Check sheet for the modelled part. Datum: model origin and axes. Units: mm. Give positions to 0.01 mm unless a question says otherwise; leave off trailing zeros. Write each loop counter-clockwise with the first axis right and the second up, starting at its lowest first coordinate (ties: lowest second). Pieces come first, ordered by that corner, then holes. Notation, with made-up numbers: (86, 72) -> (93, 72) arc R14 ccw to (93, 96) -> close; hole circle Ø9 at (31, -1). An arc over 180 degrees is marked (long way). Answer as a JSON object with one key per item and string values.
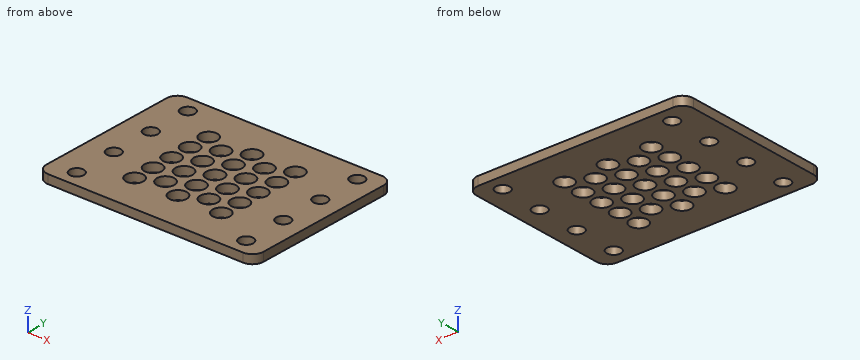
from build123d import *

# Parameters (mm, degrees)
SKETCH_W     = 100
SKETCH_H     = 75
SKETCH_R     = 3.2
PAD_DEPTH    = 4
SKETCH001_R  = 4
POCKET_DEPTH = 5
FILLET_R     = 5


with BuildPart() as part:
    # Sketch → Pad (new body)
    with BuildSketch(Plane.XY):
        with Locations((50, 37.5)):
            Rectangle(SKETCH_W, SKETCH_H)
        with Locations((11.871567, 67.5)):
            Circle(SKETCH_R, mode=Mode.SUBTRACT)
        with Locations((11.871567, 47.5)):
            Circle(SKETCH_R, mode=Mode.SUBTRACT)
        with Locations((11.871567, 27.5)):
            Circle(SKETCH_R, mode=Mode.SUBTRACT)
        with Locations((11.871567, 7.5)):
            Circle(SKETCH_R, mode=Mode.SUBTRACT)
        with Locations((90, 67.5)):
            Circle(SKETCH_R, mode=Mode.SUBTRACT)
        with Locations((90, 47.5)):
            Circle(SKETCH_R, mode=Mode.SUBTRACT)
        with Locations((90, 27.5)):
            Circle(SKETCH_R, mode=Mode.SUBTRACT)
        with Locations((90, 7.5)):
            Circle(SKETCH_R, mode=Mode.SUBTRACT)
    extrude(amount=PAD_DEPTH)

    # Sketch001 (on Face14 of Pad) → Pocket (cut)
    with BuildSketch(Plane.XY.offset(4)):
        with Locations((30, 57.5)):
            Circle(SKETCH001_R)
        with Locations((30, 47.5)):
            Circle(SKETCH001_R)
        with Locations((30, 37.5)):
            Circle(SKETCH001_R)
        with Locations((30, 27.5)):
            Circle(SKETCH001_R)
        with Locations((30, 17.5)):
            Circle(SKETCH001_R)
        with Locations((50, 57.5)):
            Circle(SKETCH001_R)
        with Locations((50, 47.5)):
            Circle(SKETCH001_R)
        with Locations((50, 37.5)):
            Circle(SKETCH001_R)
        with Locations((50, 27.5)):
            Circle(SKETCH001_R)
        with Locations((50, 17.5)):
            Circle(SKETCH001_R)
        with Locations((70, 57.5)):
            Circle(SKETCH001_R)
        with Locations((70, 47.5)):
            Circle(SKETCH001_R)
        with Locations((70, 37.5)):
            Circle(SKETCH001_R)
        with Locations((70, 27.5)):
            Circle(SKETCH001_R)
        with Locations((70, 17.5)):
            Circle(SKETCH001_R)
        with Locations((40, 52.5)):
            Circle(SKETCH001_R)
        with Locations((40, 42.5)):
            Circle(SKETCH001_R)
        with Locations((40, 32.5)):
            Circle(SKETCH001_R)
        with Locations((40, 22.5)):
            Circle(SKETCH001_R)
        with Locations((60, 52.5)):
            Circle(SKETCH001_R)
        with Locations((60, 42.5)):
            Circle(SKETCH001_R)
        with Locations((60, 32.5)):
            Circle(SKETCH001_R)
        with Locations((60, 22.5)):
            Circle(SKETCH001_R)
    extrude(amount=-POCKET_DEPTH, mode=Mode.SUBTRACT)

    # Fillet
    fillet_edges = [part.edges().sort_by_distance(p)[0] for p in [
        (100, 75, 2),
        (100, 0, 2),
        (0, 75, 2),
        (0, 0, 2),
    ]]
    fillet(fillet_edges, radius=FILLET_R)


solid = part.part
1. Sectioned sample at A-A, the plane x = 60. Enter the section's corners in (y, z).
Determined:
{"outline": "(0, 0) -> (18.5, 0) -> (18.5, 4) -> (0, 4) -> close; (26.5, 0) -> (28.5, 0) -> (28.5, 4) -> (26.5, 4) -> close; (36.5, 0) -> (38.5, 0) -> (38.5, 4) -> (36.5, 4) -> close; (46.5, 0) -> (48.5, 0) -> (48.5, 4) -> (46.5, 4) -> close; (56.5, 0) -> (75, 0) -> (75, 4) -> (56.5, 4) -> close"}
2. Go/stop test with a flat-tipped pin: P1, Ø9, axis at x = 60, y = 22.5, coming from the +Z side. Record where the tip stops, or that it passes through.
Determined:
{"P1": "z = 4"}
3. Sectioned sample at B-B, the plane y = 67.5. Enter the section's corners in (x, z).
Determined:
{"outline": "(0, 0) -> (8.67, 0) -> (8.67, 4) -> (0, 4) -> close; (15.07, 0) -> (86.8, 0) -> (86.8, 4) -> (15.07, 4) -> close; (93.2, 0) -> (100, 0) -> (100, 4) -> (93.2, 4) -> close"}
4. Scan lines: L1, parallel to Y at x = 70, z = 2.1; L2, parallel to Y at x = 90, z = 1.6; L3, parallel to Y at x = 60, z = 2.1. Record each from-to range of solid material in increasing order. Write a range as [from, to].
Determined:
{"L1": "[0, 13.5], [21.5, 23.5], [31.5, 33.5], [41.5, 43.5], [51.5, 53.5], [61.5, 75]", "L2": "[0, 4.3], [10.7, 24.3], [30.7, 44.3], [50.7, 64.3], [70.7, 75]", "L3": "[0, 18.5], [26.5, 28.5], [36.5, 38.5], [46.5, 48.5], [56.5, 75]"}
5. Sectioned sample at C-C, the plane z = 3.05. State how many separate pieces and enclosed holes the cut face has, plus the area to 3 significant figures.
Determined:
{"separate pieces": "1", "enclosed holes": "31", "area": "6,070 mm^2"}
